```python
from build123d import *

# Parameters (mm, degrees)
REVOLVE1_ANGLE     = 56
SKETCH2_R          = 152.4
CUT_EXTRUDE1_DEPTH = 309.88


with BuildPart() as part:
    # Sketch1 → Revolve1 (revolve)
    with BuildSketch(Plane.XY):
        with BuildLine():
            Line((29.137194784, 179.160976849), (39.542245278, 147.180742077))
            ThreePointArc((39.542245278, 147.180742077), (38.630482432, 147.422677452), (37.717239544, 147.658964649))
            Line((37.717239544, 147.658964649), (27.627587493, 178.669812847))
            ThreePointArc((27.627587493, 178.669812847), (23.462294361, 185.748899875), (16.703713988, 190.41631151))
            ThreePointArc((16.703713988, 190.41631151), (0, 193.690277018), (-16.703713988, 190.41631151))
            ThreePointArc((-16.703713988, 190.41631151), (-23.462294361, 185.748899875), (-27.627587493, 178.669812847))
            Line((-27.627587493, 178.669812847), (-37.717239544, 147.658964649))
            ThreePointArc((-37.717239544, 147.658964649), (-38.630482432, 147.422677452), (-39.542245278, 147.180742077))
            Line((-39.542245278, 147.180742077), (-29.137194784, 179.160976849))
            ThreePointArc((-29.137194784, 179.160976849), (-24.624793891, 186.829987796), (-17.302998471, 191.886350359))
            ThreePointArc((-17.302998471, 191.886350359), (0, 195.277776974), (17.302998471, 191.886350359))
            ThreePointArc((17.302998471, 191.886350359), (24.624793891, 186.829987796), (29.137194784, 179.160976849))
        make_face()
    revolve(axis=Axis((0, 2.54, 0), (-1, 0, 0)), revolution_arc=REVOLVE1_ANGLE)

    # Sketch2 → Cut-Extrude1 (cut)
    with BuildSketch(Plane.XY):
        Circle(SKETCH2_R)
    extrude(amount=-CUT_EXTRUDE1_DEPTH, mode=Mode.SUBTRACT)


solid = part.part
```
Input: part model. Units: mm. Frame: model coordinates. A direction names the side the tool comes from. Give positions to 0.01 mm unless a question says otherwise; leave off trailing zeros. Order: outer loops, then holes, each group sorted by start corner. A loop starts at its lowest first (then second) coordinate and runs counter-clockwise, first axis right, second up. Notation, with made-up numbers: M 28,19.25 L 45,19.25 A27 cw 45,50.25 Z; hole C -0.75,8.5 d5. An arc over 180 degrees is marked long. One line per question, with ' | ' between items.
1) Access query for faces 1 (the face through (32.527, 148.888, -69.296)), 2 (the face through (32.602, 159.453, -35.33)). Directions: +Z, -Z, +X, -X, +Y, -Y. A direction counts if a zero-diameter tool reaches every point of the face in a straight line with its end or side. Return the directions, or none.
Filled in:
face 1: +Z, -Z, -Y | face 2: +Z, -Y
2) Ray query, L1, parallel to X at y = 151.5, z = -75.5; L2, parallel to X at y = 165.5, z = -88.5; L3, parallel to Y at x = 10, z = -88.5. Return the intervals inside material, ascending.
Filled in:
L1: x = -32.27 to -30.6, 30.6 to 32.27 | L2: x = -23.47 to -20.99, 20.99 to 23.47 | L3: y = 170.68 to 172.51
3) Section A-A on x = -0.5. Output: boundary loops of the cut face in (y, z), and give its area (3 significant figures).
Filled in:
outline: M 152.4,-121.2 A192.74 ccw 195.28,0 L 193.69,0 A191.15 cw 152.4,-118.66 Z | area: 206 mm2
4) Section B-B on x = -9. Output: boundary loops of the cut face in (y, z).
Filled in:
outline: M 152.13,-120.11 A191.85 ccw 194.39,0 L 192.77,0 A190.23 cw 152.13,-117.5 Z
5) Draft query along X for faces 3 (the face through (34.413, 158.933, -35.662)), 4 (the face through (-32.743, 159.03, -35.234)), 5 (the face through (-34.267, 159.369, -35.762)), 6 (the face through (0, 194, 0)). Return one class per face: pulls with the +X half, pulls with the -X half, needs draft (parallel to the pull), parting line crosses it, or undercut.
Filled in:
face 3: pulls with the +X half | face 4: undercut | face 5: pulls with the -X half | face 6: needs draft
6) Contact query for flat-ended pins moving along their axis: P1, Ø10, axis at y = 165, z = -105.5, coming from the +X side; P2, Ø10, axis at y = 176, z = -56.5, coming from the +X side; P3, Ø5, axis at y = 155.5, z = -22.5, coming from the +X side. Output: stop coordinate, or through.
Filled in:
P1: stops at x = 18.71 | P2: stops at x = 28.86 | P3: stops at x = 37.11
